Geometry check sheet. Reference: drawing and pictorial views, mm from the part's lowest x, y, z. Round coordinates to 2 decimals unless told otherwise and drop trailing zeros. Loops run counter-clockwise (first coordinate to the right, second up) from the corner with the lowest first, then second, coordinate; pieces in that order, holes last. Notation, with made-up numbers: (-32, 30.5) - (10, 30.5) arc R17 ccw to (10, 55.5) - close; hole circle Ø9 at (41.5, -18). An arc over 180 degrees is marked (long way). Answer in a Markdown table with one row per item. Add a question column.
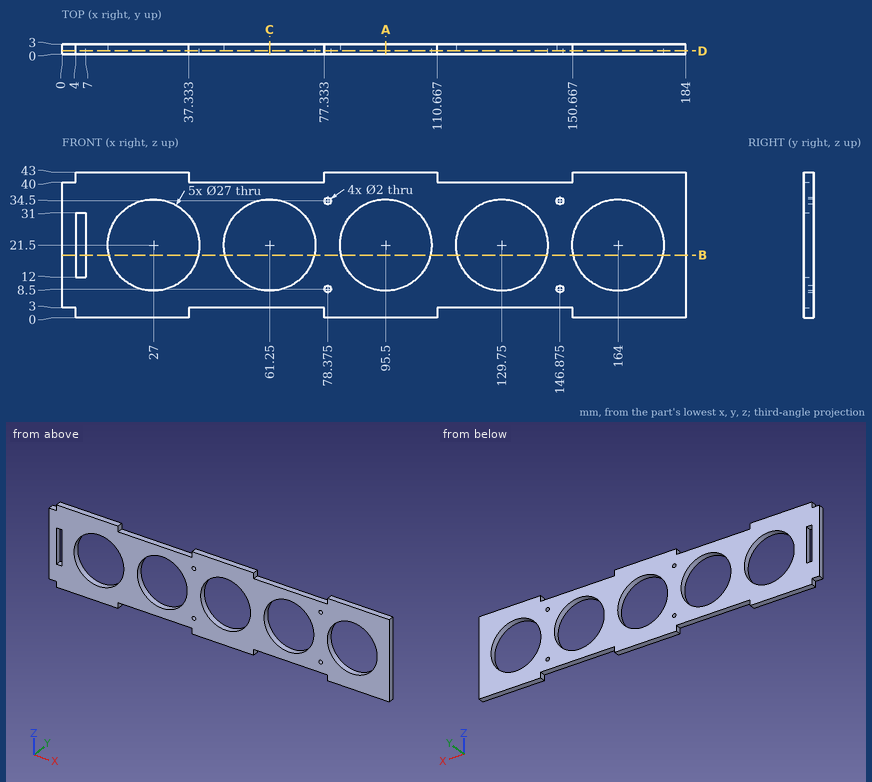
Q1. Cross-section at C-C, the plane x = 61.25. Enter the section's corners in (y, z), plus the area to 3 significant figures.
Q2. Cross-section at B-B, the plane z = 18.5. Enter the section's corners in (x, y).
Q3. Depth check by flat-ended pin: P1, Ø0.9, axis at x = 121, y = 1.5, coming from the -Z side; P2, Ø1.5, axis at y = 1, z = 42, coming from the -X side. Enter the tip coordinate at first touch or a pass-through.
Q4. Cross-section at D-D, the plane y = 1. State how many separate pieces and enclosed holes the cut face has.
Q5. Scan lines: line 1 (Z direction, x = 95.5, y = 1.2); line 2 (X direction, y = 2.45, z = 11.5); line 3 (Z direction, x = 78, y = 2.9). Record each from-to range of solid material in increasing order. Write a range as from..to.
Q6. Cross-section at A-A, the plane x = 95.5. Enter the section's corners in (y, z).
Check sheet entries:
| question | item | result |
|---|---|---|
| 1 | outline | (0, 3) - (3, 3) - (3, 8) - (0, 8) - close; (0, 35) - (3, 35) - (3, 40) - (0, 40) - close |
| 1 | area | 30.0 mm² |
| 2 | outline | (0, 0) - (4, 0) - (4, 3) - (0, 3) - close; (7, 0) - (13.84, 0) - (13.84, 3) - (7, 3) - close; (40.16, 0) - (48.09, 0) - (48.09, 3) - (40.16, 3) - close; (74.41, 0) - (82.34, 0) - (82.34, 3) - (74.41, 3) - close; (108.66, 0) - (116.59, 0) - (116.59, 3) - (108.66, 3) - close; (142.91, 0) - (150.84, 0) - (150.84, 3) - (142.91, 3) - close; (177.16, 0) - (184, 0) - (184, 3) - (177.16, 3) - close |
| 3 | P1 | z = 3 |
| 3 | P2 | x = 4 |
| 4 | separate pieces | 1 |
| 4 | enclosed holes | 10 |
| 5 | line 1 | 0..8, 35..43 |
| 5 | line 2 | 0..17.93, 36.07..52.18, 70.32..86.43, 104.57..120.68, 138.82..154.93, 173.07..184 |
| 5 | line 3 | 0..7.57, 9.43..33.57, 35.43..43 |
| 6 | outline | (0, 0) - (3, 0) - (3, 8) - (0, 8) - close; (0, 35) - (3, 35) - (3, 43) - (0, 43) - close |
